```python
from build123d import *

# Parameters (mm, degrees)
RESSALTO_EXTRUS_O1_DEPTH = 60
ESBO_O2_W                = 40
ESBO_O2_H                = 44
CORTE_EXTRUS_O1_DEPTH    = 66
CORTE_EXTRUS_O3_REACH    = 62
ESBO_O4_R                = 2
ESBO_O5_R                = 27.5
CORTE_EXTRUS_O4_DEPTH    = 5
ESBO_O6_R                = 2
CORTE_EXTRUS_O5_DEPTH    = 10
FILETE2_R                = 6


with BuildPart() as part:
    # Esboço1 → Ressalto-extrusão1 (new body)
    with BuildSketch(Plane.XY):
        Polygon((0, 0), (4, 0), (4, 56), (65, 56), (65, 60), (0, 60), align=None)
    extrude(amount=RESSALTO_EXTRUS_O1_DEPTH)

    # Esboço2 → Corte-extrusão1 (cut, through all)
    with BuildSketch(Plane.ZY):
        with Locations((30, 30)):
            Rectangle(ESBO_O2_W, ESBO_O2_H)
    extrude(amount=-CORTE_EXTRUS_O1_DEPTH, mode=Mode.SUBTRACT)

    # Esboço4 → Corte-extrusão3 (cut, up to next)
    with BuildSketch(Plane.ZX.offset(60), mode=Mode.PRIVATE) as corte_extrus_o3_sk1:
        with Locations((5, 60)):
            Circle(ESBO_O4_R)
    corte_extrus_o3_tool1 = extrude(corte_extrus_o3_sk1.sketch, amount=-CORTE_EXTRUS_O3_REACH, mode=Mode.PRIVATE) & part.part
    add(corte_extrus_o3_tool1.solids().sort_by_distance((60, 60, 5))[0], mode=Mode.SUBTRACT)
    # Esboço4 → Corte-extrusão3 (cut, up to next)
    with BuildSketch(Plane.ZX.offset(60), mode=Mode.PRIVATE) as corte_extrus_o3_sk2:
        with Locations((55, 60)):
            Circle(ESBO_O4_R)
    corte_extrus_o3_tool2 = extrude(corte_extrus_o3_sk2.sketch, amount=-CORTE_EXTRUS_O3_REACH, mode=Mode.PRIVATE) & part.part
    add(corte_extrus_o3_tool2.solids().sort_by_distance((60, 60, 55))[0], mode=Mode.SUBTRACT)
    # Esboço4 → Corte-extrusão3 (cut, up to next)
    with BuildSketch(Plane.ZX.offset(60), mode=Mode.PRIVATE) as corte_extrus_o3_sk3:
        with Locations((5, 10)):
            Circle(ESBO_O4_R)
    corte_extrus_o3_tool3 = extrude(corte_extrus_o3_sk3.sketch, amount=-CORTE_EXTRUS_O3_REACH, mode=Mode.PRIVATE) & part.part
    add(corte_extrus_o3_tool3.solids().sort_by_distance((10, 60, 5))[0], mode=Mode.SUBTRACT)
    # Esboço4 → Corte-extrusão3 (cut, up to next)
    with BuildSketch(Plane.ZX.offset(60), mode=Mode.PRIVATE) as corte_extrus_o3_sk4:
        with Locations((55, 10)):
            Circle(ESBO_O4_R)
    corte_extrus_o3_tool4 = extrude(corte_extrus_o3_sk4.sketch, amount=-CORTE_EXTRUS_O3_REACH, mode=Mode.PRIVATE) & part.part
    add(corte_extrus_o3_tool4.solids().sort_by_distance((10, 60, 55))[0], mode=Mode.SUBTRACT)

    # Esboço5 → Corte-extrusão4 (cut, through all)
    with BuildSketch(Plane(origin=(0, 56, 0), x_dir=(0, 0, -1), z_dir=(0, -1, 0))):
        with Locations((-30, 35)):
            Circle(ESBO_O5_R)
    extrude(amount=-CORTE_EXTRUS_O4_DEPTH, mode=Mode.SUBTRACT)

    # Esboço6 → Corte-extrusão5 (cut)
    with BuildSketch(Plane.ZY):
        with Locations((6, 6)):
            Circle(ESBO_O6_R)
        with Locations((54, 6)):
            Circle(ESBO_O6_R)
    extrude(amount=-CORTE_EXTRUS_O5_DEPTH, mode=Mode.SUBTRACT)

    # Filete2
    filete2_edges = [part.edges().sort_by_distance(p)[0] for p in [
        (0, 60, 30),
        (65, 58, 60),
        (65, 58, 0),
        (2, 0, 60),
        (2, 0, 0),
    ]]
    fillet(filete2_edges, radius=FILETE2_R)


solid = part.part
```
Read the model definition and answer for the solid it produces. Units are mm, in the model's axes. A direction names the side the tool comes from. Give positions to 0.01 mm unless a question says otherwise; leave off trailing zeros. Order: outer loops, then holes, each group sorted by start corner. A loop starts at its lowest first (then second) coordinate and runs counter-clockwise, first axis right, second up.
(1) Given pin 1 (18 mm diameter, centred on x = 46.5, z = 26.5, fed in from -Y); pin 2 (6.5 mm diameter, centred on x = 60, z = 55, fed in from -Y); pin 3 (2 mm diameter, centred on x = 1.5, z = 30.5, fed in from +Y); pin 4 (4.5 mm diameter, centred on x = 10, z = 5, fed in from +Y), each flat-ended and moving along its own axis, determine where each tip first touches the part or whether it passes through.
(2) For a pull along X with two mould halves and no side action, classify faces 1 (the flat face through (2, 30, 50)), 2 (the cylindrical face through (62, 58, 55)), 3 (the flat face through (65, 58, 30)) as released by +X, released by -X, zero draft, split by the parting line, or undercut.
(3) For faces 4 (the flat face through (4, 27.6, 9.6)), 5 (the flat face through (2, 8, 30)), 6 (the flat face through (0, 21.4, 9.6)), determine the directions among +Z, -Z, +X, -X, +Y, -Y from which every point of the face is accessible in a straight line to the end or side of a thin tool.
(4) Find section A-A (z = 30). Give the vertices of the cut face in (x, y).
(5) Straight lines are drawn through the part: L1, parallel to X at y = 58, z = 55; L2, parallel to X at y = 57.2, z = 55; L3, parallel to Y at x = 8, z = 47. For each, find the intervals that lie inside material, in ascending order.
(6) Find section C-C (y = 11). Give the vertices of the cut face in (x, z).
(7) Find section D-D (x = 60). Give the vertices of the cut face in (y, z), plus the area to 3 significant figures.
(8) Find section B-B (x = 51.5). Give the vertices of the cut face in (y, z), plus the area to 3 significant figures.
Result sheet:
1. pin 1: passes through
1. pin 2: stops at y = 56
1. pin 3: stops at y = 58.87
1. pin 4: stops at y = 60
2. face 1: zero draft
2. face 2: undercut
2. face 3: released by +X
3. face 4: +Z, -Z, +X, -Y
3. face 5: +X, -X
3. face 6: +Z, -Z, -X, +Y, -Y
4. outline: (0, 0) - (4, 0) - (4, 8) - (0, 8) - close; (0, 52) - (4, 52) - (4, 56) - (7.5, 56) - (7.5, 60) - (6, 60) arc R6 ccw to (0, 54) - close; (62.5, 56) - (65, 56) - (65, 60) - (62.5, 60) - close
5. L1: x = 1.53 to 8, 12 to 23.54, 46.46 to 58, 62 to 64.92
5. L2: x = 0.92 to 8, 12 to 23.54, 46.46 to 58, 62 to 64.92
5. L3: y = 56 to 60
6. outline: (0, 0) - (4, 0) - (4, 10) - (0, 10) - close; (0, 50) - (4, 50) - (4, 60) - (0, 60) - close
7. outline: (56, 0.08) - (60, 0.08) - (60, 3) - (56, 3) - close; (56, 7) - (60, 7) - (60, 18.54) - (56, 18.54) - close; (56, 41.46) - (60, 41.46) - (60, 53) - (56, 53) - close; (56, 57) - (60, 57) - (60, 59.92) - (56, 59.92) - close
7. area: 116 mm2
8. outline: (56, 0) - (60, 0) - (60, 8) - (56, 8) - close; (56, 52) - (60, 52) - (60, 60) - (56, 60) - close
8. area: 64.0 mm2
